The model under review builds one solid part; all positions refer to its coordinate system, in mm. A direction names the side the tool comes from. Round coordinates to 2 decimals unless told otherwise and drop trailing zeros. Loops run counter-clockwise (first coordinate to the right, second up) from the corner with the lowest first, then second, coordinate; pieces in that order, holes last. Notation, with made-up numbers: M 8,76 L 21,76 A28 ccw 21,96 Z; hole C -40,-36 d5. An arc over 180 degrees is marked long. Answer in a Markdown table with one row per item. Add a question column.
Autodesk Inventor part; units mm, degrees
ref_plane "Work Plane1" through (0, 2.2, 0) normal (0, 1, 0) x (1, 0, 0)
ref_plane "Work Plane2" through (-19.708, -2.44, -51.7905) normal (0, 1, 0) x (0, 0, 1)
ref_plane "YZ Plane" through (0, 0, 0) normal (1, 0, 0) x (0, 1, 0)
sketch "Sketch1" plane through (0, 0, 0) normal (0, 1, 0) x (-1, 0, 0)
  line L0 (16.25, 21) -> (-16.25, 21)
  line L1 (-17.05, 20.2) -> (-17.05, -20.2)
  line L2 (-16.25, -21) -> (16.25, -21)
  line L3 (17.05, -20.2) -> (17.05, 20.2)
  line L4 (17.05, 21) -> (-17.05, -21) construction
  line L5 (-17.05, 21) -> (17.05, -21) construction
  line L6 (16.25, 21) -> (17.05, 20.2)
  line L7 (17.05, -20.2) -> (16.25, -21)
  line L8 (-16.25, -21) -> (-17.05, -20.2)
  line L9 (-17.05, 20.2) -> (-16.25, 21)
  point P0 (0, 0)
  dimension "d0" = 34.1
  dimension "d1" = 42
  dimension "d4" = 0.8
  dimension "d5" = 0.8
  dimension "d6" = 0.8
  dimension "d7" = 0.8
  dimension "d8" = 0.8
  dimension "d9" = 0.8
  dimension "d10" = 0.8
  dimension "d11" = 0.8
extrude "Extrusion1" add sketch "Sketch1" along normal blind 1.2
ref_plane "Work Plane1" through (0, 2.2, 0) normal (0, 1, 0) x (1, 0, 0)
sketch "Sketch2" plane through (0, 2.2, 0) normal (0, 1, 0) x (1, 0, 0)
  line L0 (-15.85, -17.375) -> (15.85, -17.375)
  line L1 (15.85, -17.375) -> (15.85, 17.675)
  line L2 (15.85, 17.675) -> (-15.85, 17.675)
  line L3 (-15.85, 17.675) -> (-15.85, -17.375)
  line L4 (-15.85, -17.375) -> (15.85, 17.675) construction
  line L5 (15.85, -17.375) -> (-15.85, 17.675) construction
  point P0 (0, 0.15)
  dimension "d13" = 31.7
  dimension "d14" = 35.05
extrude "Extrusion2" add sketch "Sketch2" along normal blind 1.8
sketch "Sketch3" plane through (0, 4, 0) normal (0, 1, 0) x (1, 0, 0)
  line L0 (-15.85, -17.375) -> (15.85, -17.375)
  line L1 (15.85, -17.375) -> (15.85, 17.675)
  line L2 (15.85, 17.675) -> (-15.85, 17.675)
  line L3 (-15.85, 17.675) -> (-15.85, -17.375)
  line L4 (-15.65, -17.175) -> (15.65, -17.175)
  line L5 (15.65, -17.175) -> (15.65, 17.475)
  line L6 (15.65, 17.475) -> (-15.65, 17.475)
  line L7 (-15.65, 17.475) -> (-15.65, -17.175)
  point P0 (0, 0)
  dimension "d17" = 0.2
extrude "Extrusion3" add sketch "Sketch3" along normal blind 0.1
sketch "Sketch4" plane through (0, 1.2, 0) normal (0, 1, 0) x (1, 0, 0)
  line L0 (-14, -10) -> (14, -10)
  line L1 (14, -10) -> (14, 10)
  line L2 (14, 10) -> (-14, 10)
  line L3 (-14, 10) -> (-14, -10)
  line L4 (-14, -10) -> (14, 10) construction
  line L5 (14, -10) -> (-14, 10) construction
  point P0 (0, 0)
  dimension "d20" = 28
  dimension "d21" = 20
extrude "Extrusion4" add sketch "Sketch4" along normal up to surface (1 mm away)
sketch "Sketch5" plane through (0, 0, 0) normal (0, -1, 0) x (1, 0, 0)
  line L0 (15.8, -20) -> (13.86, -20)
  line L1 (13.61, -19.75) -> (13.61, -17.81)
  line L2 (13.86, -17.56) -> (15.8, -17.56)
  line L3 (16.05, -17.81) -> (16.05, -19.75)
  line L4 (16.05, -19.75) -> (15.8, -20)
  line L5 (13.86, -20) -> (13.61, -19.75)
  line L6 (13.61, -17.81) -> (13.86, -17.56)
  line L7 (15.8, -17.56) -> (16.05, -17.81)
  line L8 (13.36, -20) -> (11.42, -20)
  line L9 (11.17, -19.75) -> (11.17, -17.81)
  line L10 (11.42, -17.56) -> (13.36, -17.56)
  line L11 (13.61, -17.81) -> (13.61, -19.75)
  line L12 (13.61, -19.75) -> (13.36, -20)
  line L13 (11.42, -20) -> (11.17, -19.75)
  line L14 (11.17, -17.81) -> (11.42, -17.56)
  line L15 (13.36, -17.56) -> (13.61, -17.81)
  line L16 (10.92, -20) -> (8.98, -20)
  line L17 (8.73, -19.75) -> (8.73, -17.81)
  line L18 (8.98, -17.56) -> (10.92, -17.56)
  line L19 (11.17, -17.81) -> (11.17, -19.75)
  line L20 (11.17, -19.75) -> (10.92, -20)
  line L21 (8.98, -20) -> (8.73, -19.75)
  line L22 (8.73, -17.81) -> (8.98, -17.56)
  line L23 (10.92, -17.56) -> (11.17, -17.81)
  line L24 (8.48, -20) -> (6.54, -20)
  line L25 (6.29, -19.75) -> (6.29, -17.81)
  line L26 (6.54, -17.56) -> (8.48, -17.56)
  line L27 (8.73, -17.81) -> (8.73, -19.75)
  line L28 (8.73, -19.75) -> (8.48, -20)
  line L29 (6.54, -20) -> (6.29, -19.75)
  line L30 (6.29, -17.81) -> (6.54, -17.56)
  line L31 (8.48, -17.56) -> (8.73, -17.81)
  line L32 (6.04, -20) -> (4.1, -20)
  line L33 (3.85, -19.75) -> (3.85, -17.81)
  line L34 (4.1, -17.56) -> (6.04, -17.56)
  line L35 (6.29, -17.81) -> (6.29, -19.75)
  line L36 (6.29, -19.75) -> (6.04, -20)
  line L37 (4.1, -20) -> (3.85, -19.75)
  line L38 (3.85, -17.81) -> (4.1, -17.56)
  line L39 (6.04, -17.56) -> (6.29, -17.81)
  line L40 (3.6, -20) -> (1.66, -20)
  line L41 (1.41, -19.75) -> (1.41, -17.81)
  line L42 (1.66, -17.56) -> (3.6, -17.56)
  line L43 (3.85, -17.81) -> (3.85, -19.75)
  line L44 (3.85, -19.75) -> (3.6, -20)
  line L45 (1.66, -20) -> (1.41, -19.75)
  line L46 (1.41, -17.81) -> (1.66, -17.56)
  line L47 (3.6, -17.56) -> (3.85, -17.81)
  line L48 (1.16, -20) -> (-0.78, -20)
  line L49 (-1.03, -19.75) -> (-1.03, -17.81)
  line L50 (-0.78, -17.56) -> (1.16, -17.56)
  line L51 (1.41, -17.81) -> (1.41, -19.75)
  line L52 (1.41, -19.75) -> (1.16, -20)
  line L53 (-0.78, -20) -> (-1.03, -19.75)
  line L54 (-1.03, -17.81) -> (-0.78, -17.56)
  line L55 (1.16, -17.56) -> (1.41, -17.81)
  line L56 (-1.28, -20) -> (-3.22, -20)
  line L57 (-3.47, -19.75) -> (-3.47, -17.81)
  line L58 (-3.22, -17.56) -> (-1.28, -17.56)
  line L59 (-1.03, -17.81) -> (-1.03, -19.75)
  line L60 (-1.03, -19.75) -> (-1.28, -20)
  line L61 (-3.22, -20) -> (-3.47, -19.75)
  line L62 (-3.47, -17.81) -> (-3.22, -17.56)
  line L63 (-1.28, -17.56) -> (-1.03, -17.81)
  point P0 (16.05, -20)
  point P1 (13.61, -17.56)
  point P2 (13.61, -20)
  point P3 (16.05, -17.56)
  point P4 (13.61, -20)
  point P5 (11.17, -17.56)
  point P6 (11.17, -20)
  point P7 (13.61, -17.56)
  point P8 (11.17, -20)
  point P9 (8.73, -17.56)
  point P10 (8.73, -20)
  point P11 (11.17, -17.56)
  point P12 (8.73, -20)
  point P13 (6.29, -17.56)
  point P14 (6.29, -20)
  point P15 (8.73, -17.56)
  point P16 (6.29, -20)
  point P17 (3.85, -17.56)
  point P18 (3.85, -20)
  point P19 (6.29, -17.56)
  point P20 (3.85, -20)
  point P21 (1.41, -17.56)
  point P22 (1.41, -20)
  point P23 (3.85, -17.56)
  point P24 (1.41, -20)
  point P25 (-1.03, -17.56)
  point P26 (-1.03, -20)
  point P27 (1.41, -17.56)
  point P28 (-1.03, -20)
  point P29 (-3.47, -17.56)
  point P30 (-3.47, -20)
  point P31 (-1.03, -17.56)
  dimension "d42" = 2.44
extrude "Extrusion5" add sketch "Sketch5" along normal blind 2.44
sketch "Sketch6" plane through (0, 0, 0) normal (0, -1, 0) x (1, 0, 0)
  line L0 (-15, 8.95) -> (15, 8.95)
  line L1 (15, 8.95) -> (15, 18.95)
  line L2 (15, 18.95) -> (-15, 18.95)
  line L3 (-15, 18.95) -> (-15, 8.95)
  line L4 (-15, 8.95) -> (15, 18.95) construction
  line L5 (15, 8.95) -> (-15, 18.95) construction
  line L6 (-16.25, 21) -> (16.25, 21)
  line L7 (0, 21) -> (0, 18.95)
  point P0 (0, 0)
  point P1 (0, 18.95)
  dimension "d49" = 30
  dimension "d50" = 10
  dimension "d51" = 2.05
ref_plane "Work Plane2" through (-19.708, -2.44, -51.7905) normal (0, 1, 0) x (0, 0, 1)
extrude "Extrusion6" add sketch "Sketch6" along normal up to surface (2.44 mm away)
equation "\"d5\" = d4"
equation "\"d6\" = d4"
equation "\"d7\" = d6"
equation "\"d8\" = d4"
equation "\"d9\" = d8"
equation "\"d10\" = d4"
equation "\"d11\" = d10"
properties part number "Display"
1. Take a section at C-C, the plane z = -3.5. State the section outline as (x, y) points.
2. Mouldability with a two-part tool opening along Z and no side actions: class faces 6 (the flat face through (17.05, 1, 0)), 7 (the flat face through (3, -1, -17.56)), 8 (the flat face through (0, 1, 21)) as released by +Z, released by -Z, zero draft, split by the parting line, or undercut.
3. Take a section at B-B, the plane x = -11.5. State the section outline as (y, z) points (3 decimals), and give its area (3 significant figures).
4. For pin 1 Ø1.6 at (x, y) = (9.5, -1.5) entering from -Z; pin 2 Ø0.9 at (y, z) = (3, 6) entering from -X; pin 3 Ø1 at (x, z) = (-7.5, -10) entering from +Y, all flat-tipped, find the tip position at first contact; note any pin that passes through.
5. Take a section at A-A, the plane z = 12. State the section outline as (x, y) points, and give its area (3 significant figures).
6. Machinability: for faces 1 (the flat face through (10, -1, -17.56)), 2 (the flat face through (5, -1, -20)), 3 (the flat face through (0, 4, 0)), 4 (the flat face through (0, 2, 10)), 5 (the flat face through (16.05, -1, -19)), which of the approach directions +Z, -Z, +X, -X, +Y, -Y give a long, thin tool a straight path to every point of the face, cutting with its end or side? Answer none if there is none.
7. To check wall thickness, follow probe 1 along Y at (x, z) = (14.5, 8.5); probe 2 along Z at (x, y) = (10, -0.5); probe 3 along X at (y, z) = (1.5, -7.5). State the ranges of each line that lie inside material, in increasing order.
8. Take a section at D-D, the plane y = 3.5. State the section outline as (x, z) points (3 decimals), and give its area (3 significant figures).
Check sheet entries:
| question | item | result |
|---|---|---|
| 1 | outline | M -17.05,0 L 17.05,0 L 17.05,1.2 L 14,1.2 L 14,2.2 L 15.85,2.2 L 15.85,4.1 L 15.65,4.1 L 15.65,4 L -15.65,4 L -15.65,4.1 L -15.85,4.1 L -15.85,2.2 L -14,2.2 L -14,1.2 L -17.05,1.2 Z |
| 2 | face 6 | zero draft |
| 2 | face 7 | undercut |
| 2 | face 8 | released by +Z |
| 3 | outline | M -2.44,8.95 L 0,8.95 L 0,-21 L 1.2,-21 L 1.2,-10 L 2.2,-10 L 2.2,-17.675 L 4.1,-17.675 L 4.1,-17.475 L 4,-17.475 L 4,17.175 L 4.1,17.175 L 4.1,17.375 L 2.2,17.375 L 2.2,10 L 1.2,10 L 1.2,21 L 0,21 L 0,18.95 L -2.44,18.95 Z |
| 3 | area | 158 mm^2 |
| 4 | pin 1 | stops at z = -20 |
| 4 | pin 2 | stops at x = -15.85 |
| 4 | pin 3 | stops at y = 4 |
| 5 | outline | M -17.05,0 L -15,0 L -15,-2.44 L 15,-2.44 L 15,0 L 17.05,0 L 17.05,1.2 L -17.05,1.2 Z; M -15.85,2.2 L 15.85,2.2 L 15.85,4.1 L 15.65,4.1 L 15.65,4 L -15.65,4 L -15.65,4.1 L -15.85,4.1 Z |
| 5 | area | 171 mm^2 |
| 6 | face 1 | +X, -X, -Y |
| 6 | face 2 | -Z, +X, -X, -Y |
| 6 | face 3 | +Y |
| 6 | face 4 | +Z, +X, -X |
| 6 | face 5 | +Z, -Z, +X, -Y |
| 7 | probe 1 | y = 0 to 1.2, 2.2 to 4 |
| 7 | probe 2 | z = -20 to -17.56, 8.95 to 18.95 |
| 7 | probe 3 | x = -14 to 14 |
| 8 | outline | M -15.85,-17.675 L 15.85,-17.675 L 15.85,17.375 L -15.85,17.375 Z |
| 8 | area | 1,110 mm^2 |
